Part model, mm, in its own coordinate system. A direction names the side the tool comes from. Round coordinates to 2 decimals unless told otherwise and drop trailing zeros. Loops run counter-clockwise (first coordinate to the right, second up) from the corner with the lowest first, then second, coordinate; pieces in that order, holes last. Notation, with made-up numbers: (-11.5, 12.25) -> (38.5, 12.25) arc R27 ccw to (38.5, 40.25) -> close; hole circle Ø3 at (-17, -9). An arc over 180 degrees is marked (long way). Use a Markdown table: item, result. Add a question column.
Item 1: Cut at B-B, the plane x = -66.5. List the corners of the cut face in (y, z).
Item 2: Flat gauge pins, fed straight in: pin 1 (1 mm diameter, centred on x = -37.5, z = 1.5, fed in from +Y); pin 2 (0.8 mm diameter, centred on y = -27.5, z = 78, fed in from +X); pin 3 (8 mm diameter, centred on x = -7.5, y = 9, fed in from +Z); pin 4 (10 mm diameter, centred on x = -72.39, y = 26.67, fed in from +Z). Where does each tip first touch, or does it go through?
Item 3: Probe line 1 (X direction, y = -16, z = 9.5); line 2 (X direction, y = -28.35, z = 74.93); line 3 (Z direction, x = 4.5, y = 29). List the from-to ranges inside material, lowest first. Write a range as [from, to].
Item 4: Two-plate mould, pull along Y, no slides. Class faces 1 (the face through (-1, -31.75, 34)), 2 (the face through (11.82, 25.45, 21.22)), 3 (the face through (-35.386, -28, 8)), 4 (the face through (-63, 0, 69)): pulls with the +Y half, pulls with the -Y half, needs draft (parallel to the pull), parting line crosses it, or undercut.
Item 5: Cut at D-D, the plane x = -31.75. List the corners of the cut face in (y, z), plus the area to 3 significant figures.
Item 6: Cut at C-C, the plane z = 56.5. List the corners of the cut face in (x, y), plus the area to 3 significant figures.
Item 7: Cut at A-A, the plane y = 20. List the corners of the cut face in (x, z).
Item 8: Which spindle directions (+Z, -Z, +X, -X, +Y, -Y) get a long thin tool onto all of the face, cutting with end or side? Do faces 5 (the face through (-63.5, -16, 54)), 6 (the face through (-1.27, -2, 55)), 7 (the face through (-72, 0, 19.304)), 8 (the face through (-60.96, -30, 43)). Say none if no direction does.
```python
from build123d import *

# Parameters (mm, degrees)
SKETCH3_W                  = 63.5
SKETCH3_H                  = 86.36
BOSS_EXTRUDE2_DEPTH        = 31.75
SKETCH4_W                  = 58.42
SKETCH4_H                  = 81.28
CUT_EXTRUDE2_DEPTH         = 27.94
POWER_JACK_HOLE_REACH      = 113.796
SKETCH5_R                  = 5.715
MOTOR_MOUNTING_SHAPE_DEPTH = 63.5
MOTOR_MOUNTING_HOLES_REACH = 129.254
SKETCH8_R                  = 1.6
SKETCH13_W                 = 60.96
SKETCH13_H                 = 83.82
CUT_EXTRUDE7_DEPTH         = 3.81
SKETCH9_W                  = 15.24
SKETCH9_H                  = 15.24
BOSS_EXTRUDE3_DEPTH        = 66
CHAMFER1_SIZE              = 2
CUT_EXTRUDE5_DEPTH         = 126.858217451
SKETCH12_R                 = 3.175
LEG_HOLES_DEPTH            = 111.448682274
CHAMFER2_SIZE              = 1
BOSS_EXTRUDE5_START        = -5.08
SKETCH14_W                 = 58.42
SKETCH14_H                 = 81.28
SKETCH14_W_2               = 53.34
SKETCH14_H_2               = 76.2
BOSS_EXTRUDE5_DEPTH        = 2.54
CUT_EXTRUDE8_REACH         = 127.128
SKETCH15_R                 = 2.5
CHAMFER3_SIZE              = 1.27
SKETCH16_R                 = 1.35
BOSS_EXTRUDE6_DEPTH        = 2.54


with BuildPart() as part:
    # Sketch3 → Boss-Extrude2 (new body)
    with BuildSketch(Plane(origin=(0, 0, 0), x_dir=(-1, 0, 0), z_dir=(0, 1, 0))):
        with Locations((31.75, 43.18)):
            Rectangle(SKETCH3_W, SKETCH3_H)
    extrude(amount=-BOSS_EXTRUDE2_DEPTH)

    # Sketch4 → Cut-Extrude2 (cut)
    with BuildSketch(Plane.XZ.offset(31.75)):
        with Locations((-31.75, 43.18)):
            Rectangle(SKETCH4_W, SKETCH4_H)
    extrude(amount=-CUT_EXTRUDE2_DEPTH, mode=Mode.SUBTRACT)

    # Sketch5 → Power Jack Hole (cut, up to next)
    with BuildSketch(Plane(origin=(-63.5, 0, 0), x_dir=(0, 0, -1), z_dir=(1, 0, 0)), mode=Mode.PRIVATE) as power_jack_hole_sk1:
        with Locations(Location((-76.327, -19.177, 0), (0, 0, 180))):
            Circle(SKETCH5_R)
    power_jack_hole_tool1 = extrude(power_jack_hole_sk1.sketch, amount=POWER_JACK_HOLE_REACH, mode=Mode.PRIVATE) & part.part
    add(power_jack_hole_tool1.solids().sort_by_distance((-63.5, -19.177, 76.327))[0], mode=Mode.SUBTRACT)

    # Sketch6 → Motor Mounting Shape (add)
    with BuildSketch(Plane.ZY.offset(63.5)):
        Polygon((46.54, 0), (46.54, 36.83), (0, 36.83), (0, 34.29), (44, 34.29), (44, 0), align=None)
    extrude(amount=-MOTOR_MOUNTING_SHAPE_DEPTH)

    # Sketch8 → Motor-Mounting-Holes (cut, up to next)
    with BuildSketch(Plane(origin=(0, 36.83, 0), x_dir=(1, 0, 0), z_dir=(0, 1, 0)), mode=Mode.PRIVATE) as motor_mounting_holes_sk1:
        with Locations(Location((-47.25, -7.77, 0), (0, 0, 270))):
            Circle(SKETCH8_R)
    motor_mounting_holes_tool1 = extrude(motor_mounting_holes_sk1.sketch, amount=-MOTOR_MOUNTING_HOLES_REACH, mode=Mode.PRIVATE) & part.part
    # Sketch8 → Motor-Mounting-Holes (cut, up to next)
    with BuildSketch(Plane(origin=(0, 36.83, 0), x_dir=(1, 0, 0), z_dir=(0, 1, 0)), mode=Mode.PRIVATE) as motor_mounting_holes_sk2:
        with Locations(Location((-16.25, -7.77, 0), (0, 0, 270))):
            Circle(SKETCH8_R)
    motor_mounting_holes_tool2 = extrude(motor_mounting_holes_sk2.sketch, amount=-MOTOR_MOUNTING_HOLES_REACH, mode=Mode.PRIVATE) & part.part
    # Sketch8 → Motor-Mounting-Holes (cut, up to next)
    with BuildSketch(Plane(origin=(0, 36.83, 0), x_dir=(1, 0, 0), z_dir=(0, 1, 0)), mode=Mode.PRIVATE) as motor_mounting_holes_sk3:
        with Locations(Location((-16.25, -38.77, 0), (0, 0, 270))):
            Circle(SKETCH8_R)
    motor_mounting_holes_tool3 = extrude(motor_mounting_holes_sk3.sketch, amount=-MOTOR_MOUNTING_HOLES_REACH, mode=Mode.PRIVATE) & part.part
    # Sketch8 → Motor-Mounting-Holes (cut, up to next)
    with BuildSketch(Plane(origin=(0, 36.83, 0), x_dir=(1, 0, 0), z_dir=(0, 1, 0)), mode=Mode.PRIVATE) as motor_mounting_holes_sk4:
        with Locations(Location((-47.25, -38.77, 0), (0, 0, 270))):
            Circle(SKETCH8_R)
    motor_mounting_holes_tool4 = extrude(motor_mounting_holes_sk4.sketch, amount=-MOTOR_MOUNTING_HOLES_REACH, mode=Mode.PRIVATE) & part.part
    # Sketch8 → Motor-Mounting-Holes (cut, up to next)
    with BuildSketch(Plane(origin=(0, 36.83, 0), x_dir=(1, 0, 0), z_dir=(0, 1, 0)), mode=Mode.PRIVATE) as motor_mounting_holes_sk5:
        with BuildLine():
            Line((-40.64, 0), (-22.86, 0))
            Line((-22.86, 0), (-22.86, -23.27))
            ThreePointArc((-22.86, -23.27), (-31.75, -32.16), (-40.64, -23.27))
            Line((-40.64, -23.27), (-40.64, 0))
        make_face()
    motor_mounting_holes_tool5 = extrude(motor_mounting_holes_sk5.sketch, amount=-MOTOR_MOUNTING_HOLES_REACH, mode=Mode.PRIVATE) & part.part
    add(motor_mounting_holes_tool1.solids().sort_by_distance((-47.25, 36.83, 7.77))[0], mode=Mode.SUBTRACT)
    add(motor_mounting_holes_tool2.solids().sort_by_distance((-16.25, 36.83, 7.77))[0], mode=Mode.SUBTRACT)
    add(motor_mounting_holes_tool3.solids().sort_by_distance((-16.25, 36.83, 38.77))[0], mode=Mode.SUBTRACT)
    add(motor_mounting_holes_tool4.solids().sort_by_distance((-47.25, 36.83, 38.77))[0], mode=Mode.SUBTRACT)
    add(motor_mounting_holes_tool5.solids().sort_by_distance((-31.75, 36.83, 15.191166))[0], mode=Mode.SUBTRACT)

    # Sketch13 → Cut-Extrude7 (cut)
    with BuildSketch(Plane(origin=(0, 0, 0), x_dir=(1, 0, 0), z_dir=(0, 1, 0))):
        with Locations((-31.75, -43.18)):
            Rectangle(SKETCH13_W, SKETCH13_H)
    extrude(amount=-CUT_EXTRUDE7_DEPTH, mode=Mode.SUBTRACT)

    # Sketch9 → Boss-Extrude3 (add)
    # profile 1 of 2: a face of its own
    with BuildSketch(Plane.XZ.offset(31.75)):
        Polygon((1.27, 23.114), (-2.54, 23.114), (-2.54, 0), (1.27, 0), (20.32, 0), (20.32, 23.114), align=None)
        with Locations((8.89, 11.684)):
            Rectangle(SKETCH9_W, SKETCH9_H, mode=Mode.SUBTRACT)
    # profile 2 of 2: a face of its own
    with BuildSketch(Plane.XZ.offset(31.75)):
        Polygon((-60.96, 0), (-64.77, 0), (-83.82, 0), (-83.82, 23.114), (-64.77, 23.114), (-60.96, 23.114), align=None)
        with Locations((-72.39, 11.684)):
            Rectangle(SKETCH9_W, SKETCH9_H, mode=Mode.SUBTRACT)
    extrude(amount=-BOSS_EXTRUDE3_DEPTH)

    # Chamfer1
    chamfer1_edges = [part.edges().sort_by_distance(p)[0] for p in [
        (1.27, 34.25, 11.684),
        (8.89, 34.25, 19.304),
        (16.51, 34.25, 11.684),
        (8.89, 34.25, 4.064),
        (-72.39, 34.25, 19.304),
        (-80.01, 34.25, 11.684),
        (-72.39, 34.25, 4.064),
        (-64.77, 34.25, 11.684),
    ]]
    chamfer(chamfer1_edges, length=CHAMFER1_SIZE)

    # Sketch11 → Cut-Extrude5 (cut, through all)
    with BuildSketch(Plane(origin=(0, 0, 0), x_dir=(0, 0, -1), z_dir=(1, 0, 0))):
        Polygon((-44, 0), (-44, 34.29), (0, 34.29), (0, 36.83), (-86.36, 36.83), (-86.36, 0), align=None)
    extrude(amount=-CUT_EXTRUDE5_DEPTH, mode=Mode.SUBTRACT)

    # Sketch12 → Leg Holes (cut, through all)
    with BuildSketch(Plane.XY.offset(23.114)):
        with Locations((8.89, 26.67)):
            Circle(SKETCH12_R)
        with Locations((-72.39, 26.67)):
            Circle(SKETCH12_R)
    extrude(amount=-LEG_HOLES_DEPTH, mode=Mode.SUBTRACT)

    # Chamfer2
    chamfer2_edges = [part.edges().sort_by_distance(p)[0] for p in [
        (5.715, 26.67, 4.064),
        (5.715, 26.67, 19.304),
        (5.715, 26.67, 0),
        (5.715, 26.67, 23.114),
        (-75.565, 26.67, 19.304),
        (-75.565, 26.67, 0),
        (-75.565, 26.67, 4.064),
        (-75.565, 26.67, 23.114),
    ]]
    chamfer(chamfer2_edges, length=CHAMFER2_SIZE)

    # Sketch14 → Boss-Extrude5 (add)
    with BuildSketch(Plane.XZ.offset(31.75).offset(BOSS_EXTRUDE5_START)):
        with Locations((-31.75, 43.18)):
            Rectangle(SKETCH14_W, SKETCH14_H)
        with Locations((-31.75, 43.18)):
            Rectangle(SKETCH14_W_2, SKETCH14_H_2, mode=Mode.SUBTRACT)
    extrude(amount=BOSS_EXTRUDE5_DEPTH)

    # Sketch15 → Cut-Extrude8 (cut, up to next)
    with BuildSketch(Plane.XY.offset(86.36), mode=Mode.PRIVATE) as cut_extrude8_sk1:
        with Locations((-8.85, -16.55)):
            Circle(SKETCH15_R)
    cut_extrude8_tool1 = extrude(cut_extrude8_sk1.sketch, amount=-CUT_EXTRUDE8_REACH, mode=Mode.PRIVATE) & part.part
    add(cut_extrude8_tool1.solids().sort_by_distance((-8.85, -16.55, 86.36))[0], mode=Mode.SUBTRACT)

    # Chamfer3
    chamfer3_edges = [part.edges().sort_by_distance(p)[0] for p in [
        (20.32, 1.25, 0),
        (-2.54, 17.125, 0),
        (0, -15.875, 23.114),
        (-2.54, 15.22, 23.114),
        (20.32, 1.25, 23.114),
        (-60.96, 17.125, 0),
        (-60.96, 15.22, 23.114),
        (-63.5, -15.875, 23.114),
        (-83.82, 1.25, 0),
        (-83.82, 1.25, 23.114),
        (0, -15.875, 86.36),
        (-63.5, -15.875, 86.36),
    ]]
    chamfer(chamfer3_edges, length=CHAMFER3_SIZE - 0.0001)  # a hair under: the kernel refuses the full size

    # Sketch16 → Boss-Extrude6 (add)
    # profile 1 of 2: a face of its own
    with BuildSketch(Plane.XZ.offset(29.21)):
        with BuildLine():
            Line((-35.386, 2.54), (-28.114, 2.54))
            Line((-28.114, 2.54), (-28.114, 11.43))
            ThreePointArc((-28.114, 11.43), (-31.75, 15.066), (-35.386, 11.43))
            Line((-35.386, 11.43), (-35.386, 2.54))
        make_face()
        with Locations(Location((-31.75, 11.43, 0), (0, 0, 270))):
            Circle(SKETCH16_R, mode=Mode.SUBTRACT)
    # profile 2 of 2: a face of its own
    with BuildSketch(Plane.XZ.offset(29.21)):
        with BuildLine():
            Line((-35.386, 74.93), (-35.386, 83.82))
            Line((-35.386, 83.82), (-28.114, 83.82))
            Line((-28.114, 83.82), (-28.114, 74.93))
            ThreePointArc((-28.114, 74.93), (-31.75, 71.294), (-35.386, 74.93))
        make_face()
        with Locations(Location((-31.75, 74.93, 0), (0, 0, 270))):
            Circle(SKETCH16_R, mode=Mode.SUBTRACT)
    extrude(amount=-BOSS_EXTRUDE6_DEPTH)


solid = part.part
```
A:
| question | item | result |
|---|---|---|
| 1 | outline | (-31.75, 0) -> (34.25, 0) -> (34.25, 2.06) -> (32.25, 4.06) -> (-31.75, 4.06) -> close; (-31.75, 19.3) -> (32.25, 19.3) -> (34.25, 21.3) -> (34.25, 23.11) -> (-31.75, 23.11) -> close |
| 2 | pin 1 | stops at y = 0 |
| 2 | pin 2 | stops at x = 0 |
| 2 | pin 3 | passes through |
| 2 | pin 4 | stops at z = 23.11 |
| 3 | line 1 | x = [-83.82, -80.01], [-64.77, -60.96], [-2.54, 1.27], [16.51, 20.32] |
| 3 | line 2 | x = [-63.5, -58.42], [-35.39, -33.1], [-30.4, -28.11], [-5.08, 0] |
| 3 | line 3 | z = [0, 4.06], [19.3, 23.11] |
| 4 | face 1 | pulls with the -Y half |
| 4 | face 2 | undercut |
| 4 | face 3 | needs draft |
| 4 | face 4 | pulls with the +Y half |
| 5 | outline | (-31.75, 0) -> (0, 0) -> (0, 1.27) -> (-3.81, 1.27) -> (-3.81, 2.54) -> (-26.67, 2.54) -> (-26.67, 10.08) -> (-29.21, 10.08) -> (-29.21, 2.54) -> (-31.75, 2.54) -> close; (-31.75, 83.82) -> (-29.21, 83.82) -> (-29.21, 76.28) -> (-26.67, 76.28) -> (-26.67, 83.82) -> (-3.81, 83.82) -> (-3.81, 85.09) -> (0, 85.09) -> (0, 86.36) -> (-31.75, 86.36) -> close; (-29.21, 12.78) -> (-26.67, 12.78) -> (-26.67, 15.07) -> (-29.21, 15.07) -> close; (-29.21, 71.29) -> (-26.67, 71.29) -> (-26.67, 73.58) -> (-29.21, 73.58) -> close |
| 5 | area | 202 mm^2 |
| 6 | outline | (-63.5, -31.75) -> (-60.96, -31.75) -> (-60.96, -29.21) -> (-58.42, -29.21) -> (-58.42, -26.67) -> (-60.96, -26.67) -> (-60.96, -3.81) -> (-62.23, -3.81) -> (-62.23, 0) -> (-63.5, 0) -> close; (-5.08, -29.21) -> (-2.54, -29.21) -> (-2.54, -31.75) -> (0, -31.75) -> (0, 0) -> (-1.27, 0) -> (-1.27, -3.81) -> (-2.54, -3.81) -> (-2.54, -26.67) -> (-5.08, -26.67) -> close |
| 6 | area | 165 mm^2 |
| 7 | outline | (-83.82, 1.27) -> (-82.55, 0) -> (-62.23, 0) -> (-60.96, 1.27) -> (-60.96, 21.84) -> (-62.23, 23.11) -> (-82.55, 23.11) -> (-83.82, 21.84) -> close; (-2.54, 1.27) -> (-1.27, 0) -> (19.05, 0) -> (20.32, 1.27) -> (20.32, 21.84) -> (19.05, 23.11) -> (-1.27, 23.11) -> (-2.54, 21.84) -> close; hole (-80.01, 4.06) -> (-64.77, 4.06) -> (-64.77, 19.3) -> (-80.01, 19.3) -> close; hole (1.27, 4.06) -> (16.51, 4.06) -> (16.51, 19.3) -> (1.27, 19.3) -> close |
| 8 | face 5 | +Z, -X, +Y, -Y |
| 8 | face 6 | +Y |
| 8 | face 7 | +Y, -Y |
| 8 | face 8 | -Y |
